Check sheet for the modelled part. Datum: model origin and axes. Units: mm. A direction names the side the tool comes from. Round coordinates to 2 decimals unless told otherwise and drop trailing zeros. Write each loop counter-clockwise with the first axis right and the second up, starting at its lowest first coordinate (ties: lowest second). Pieces come first, ordered by that corner, then holes. Notation, with made-up numbers: M -12.5,-13.75 L 21.5,-13.75 A24 cw 21.5,25.25 Z; hole C 38.5,88.25 d10. An arc over 180 degrees is marked long. Answer in a Markdown table with one row per item.
```python
from build123d import *

# Parameters (mm, degrees)
BOSS_EXTRUDE1_DEPTH   = 29
FILLET1_R             = 5
CUT_EXTRUDE1_REACH    = 108.522
SKETCH3_W             = 196.5
SKETCH3_H             = 21
M4_CLEARANCE_HOLE1_D  = 4.5
F_4_0MM_DOWEL_HOLE1_D = 4


with BuildPart() as part:
    # Sketch2 → Boss-Extrude1 (new body)
    with BuildSketch(Plane(origin=(0, 0, 0), x_dir=(1, 0, 0), z_dir=(0, 1, 0))):
        Polygon((0, 97.9), (28, 97.9), (28, -98.6), (0, -98.6), (0, -63.45), (21, -63.45), (21, 61.6), (0, 61.6), align=None)
    extrude(amount=BOSS_EXTRUDE1_DEPTH)

    # Fillet1
    fillet1_edges = [part.edges().sort_by_distance(p)[0] for p in [
        (0, 14.5, -97.9),
        (0, 14.5, 98.6),
        (0, 14.5, 63.45),
        (21, 14.5, 63.45),
        (21, 14.5, -61.6),
        (0, 14.5, -61.6),
    ]]
    fillet(fillet1_edges, radius=FILLET1_R)

    # Cut-Extrude1: up to this face of the body (flat: up to its plane)
    cut_extrude1_end = Plane(part.part.faces().sort_by_distance((21, 14.5, 0.925))[0])
    # Sketch3 → Cut-Extrude1 (cut, up to the picked face)
    with BuildSketch(Plane.ZY, mode=Mode.PRIVATE) as cut_extrude1_sk1:
        with Locations((0.35, 14.5)):
            Rectangle(SKETCH3_W, SKETCH3_H)
    cut_extrude1_tool1 = split(extrude(cut_extrude1_sk1.sketch, amount=-CUT_EXTRUDE1_REACH, mode=Mode.PRIVATE), bisect_by=cut_extrude1_end, keep=Keep.BOTH, mode=Mode.PRIVATE)
    add(cut_extrude1_tool1.solids().sort_by(Axis((0, 14.5, 0.35), (1, 0, 0)))[0], mode=Mode.SUBTRACT)

    # M4 Clearance Hole1 (through all)
    with Locations(Plane(origin=(0, 0, 0), x_dir=(-1, 0, 0), z_dir=(0, -1, 0))):
        with Locations((-10.15, 87.9), (-10.15, 71.6), (-10.4, -73.45), (-10.4, -88.6)):
            Hole(M4_CLEARANCE_HOLE1_D / 2)

    # Ø4.0mm Dowel Hole1 (through all)
    with Locations(Plane.ZY.offset(-21)):
        with Locations((65.35, 14.5), (-34.65, 14.5), (-64.65, 14.5), (35.35, 14.5)):
            Hole(F_4_0MM_DOWEL_HOLE1_D / 2)


solid = part.part
```
1. Section check B-B, the plane z = -87.9. Record the cut outline in (x, y).
Found:
| item | result |
|---|---|
| outline | M 0,0 L 7.9,0 L 7.9,4 L 0,4 Z; M 0,25 L 7.9,25 L 7.9,29 L 0,29 Z; M 12.4,0 L 28,0 L 28,29 L 12.4,29 L 12.4,25 L 21,25 L 21,4 L 12.4,4 Z |
2. Go/stop test with flat-tipped pins: pin 1 (2.5 mm diameter, centred on y = 14.5, z = 65.35, fed in from -X); pin 2 (12 mm diameter, centred on y = 25, z = 1.5, fed in from -X). Record where each tip stops, or that it passes through.
Found:
| item | result |
|---|---|
| pin 1 | passes through |
| pin 2 | stops at x = 21 |
3. Scan lines: L1, parallel to Z at x = 10.15, y = 2.65; L2, parallel to X at y = 2.35, z = -71.6; L3, parallel to Z at x = 22.5, y = 15.75. Record each from-to range of solid material in increasing order.
Found:
| item | result |
|---|---|
| L1 | z = -97.9 to -90.15, -85.65 to -73.85, -69.35 to -61.6, 63.45 to 71.21, 75.69 to 86.36, 90.84 to 98.6 |
| L2 | x = 0 to 7.9, 12.4 to 28 |
| L3 | z = -97.9 to -66.21, -63.09 to -36.21, -33.09 to 33.79, 36.91 to 63.79, 66.91 to 98.6 |
4. Section check D-D, the plane y = 23.25. Record the cut outline in (x, z).
Found:
| item | result |
|---|---|
| outline | M 21,-97.9 L 28,-97.9 L 28,98.6 L 21,98.6 Z |
5. Section check C-C, the plane x = 19.25. Record the cut outline in (y, z).
Found:
| item | result |
|---|---|
| outline | M 0,-97.9 L 4,-97.9 L 4,-60.4 L 0,-60.4 Z; M 0,62.25 L 4,62.25 L 4,98.6 L 0,98.6 Z; M 25,-97.9 L 29,-97.9 L 29,-60.4 L 25,-60.4 Z; M 25,62.25 L 29,62.25 L 29,98.6 L 25,98.6 Z |
6. Draft check along Z on faces 6 (the face through (1.43, 27.03, 64.95)), 7 (the face through (8.152, 2.028, 73.351)), 8 (the face through (0, 2, 81)), 9 (the face through (1.5, 2.03, -96.47)). Enter one of: +Z half, -Z half, draft (parallel to the pull), parting line (faces both ways), or undercut.
Found:
| item | result |
|---|---|
| face 6 | undercut |
| face 7 | undercut |
| face 8 | draft |
| face 9 | -Z half |
7. Access from +Z, -Z, +X, -X, +Y, -Y to the whole of each face (thin tool, end or side, straight path). Record for faces 1 (the face through (1.5, 27.03, -96.47)), 2 (the face through (11, 2, -61.6)), 3 (the face through (24, 0, -1)), 4 (the face through (10, 25, 83)), 5 (the face through (21, 14, 2)).
Found:
| item | result |
|---|---|
| face 1 | -Z, -X, +Y, -Y |
| face 2 | -X, +Y, -Y |
| face 3 | +Z, -Z, +X, -X, -Y |
| face 4 | +Z, -Z, -X |
| face 5 | -X |
8. Section check A-A, the plane z = 35.35. Record the cut outline in (x, y), and give its area (3 significant figures).
Found:
| item | result |
|---|---|
| outline | M 21,0 L 28,0 L 28,12.5 L 21,12.5 Z; M 21,16.5 L 28,16.5 L 28,29 L 21,29 Z |
| area | 175 mm2 |
